Input: dimensioned drawing with shaded views. Units: mm. Origin: part minimum x, y, z. Give positions to 0.01 mm unless a question says otherwise; leave off trailing zeros. Loops run counter-clockwise (first coordinate to the right, second up) from the corner with the lowest first, then second, coordinate; pieces in that order, holes last. Notation, with made-up numbers: (-15.5, -19) -> (21.5, -19) arc R31 cw to (21.5, 19) -> close; hole circle Ø5 at (78, 59). An arc over 180 degrees is marked (long way). One line per question, with ' | ' between items. Start each with the question number.
Item 1: Material intervals for line 1 along Z through (x, y) = (2.65, 37.5); line 2 along Z through (x, y) = (1.7, 20.5); line 3 along X through (y, z) = (26.5, 9), sorted ascending. Write a range as [from, to].
Item 2: Section C-C on x = 0.45. Return loops of the section in (y, z), then the cut area to 3 significant figures.
Item 3: Section B-B on x = 4.5. Return loops of the section in (y, z), then the cut area to 3 significant figures.
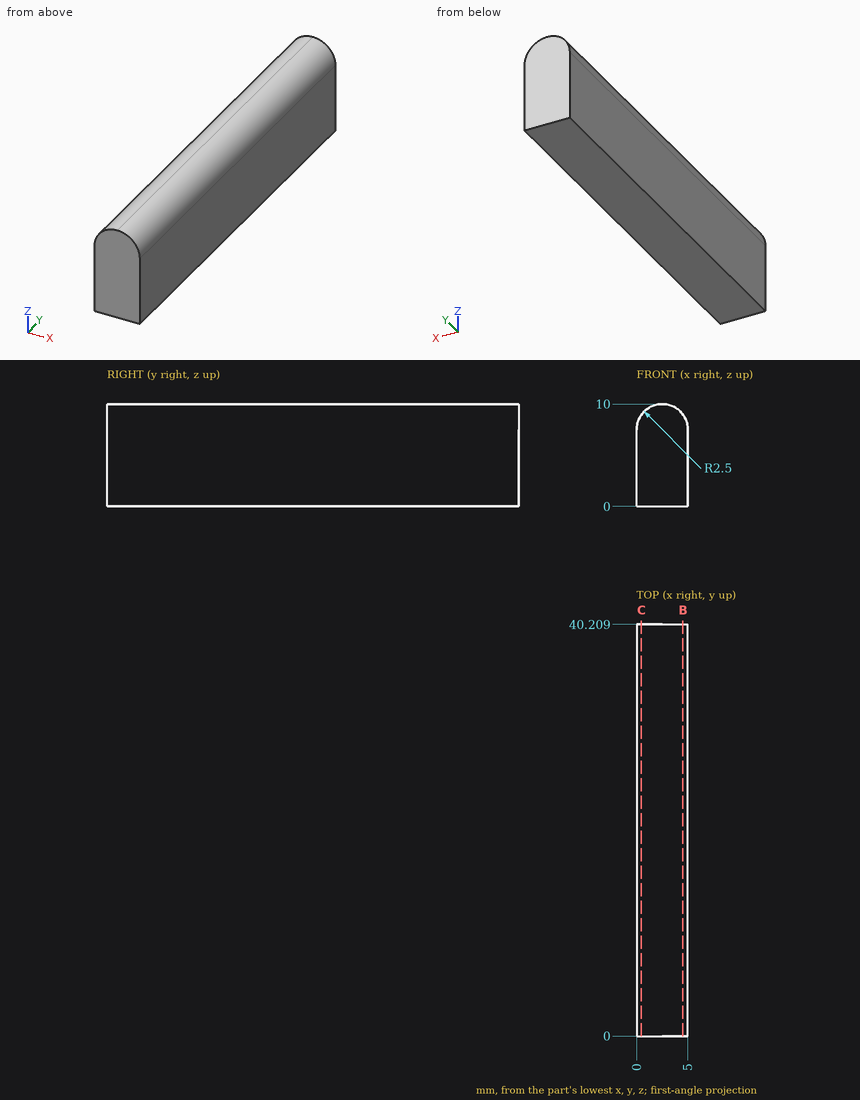
Result sheet:
1) line 1: z = [0, 10] | line 2: z = [0, 9.87] | line 3: x = [0.5, 4.5]
2) outline: (0, 0) -> (40.21, 0) -> (40.21, 8.93) -> (0, 8.93) -> close | area: 359 mm²
3) outline: (0, 0) -> (40.21, 0) -> (40.21, 9) -> (0, 9) -> close | area: 362 mm²
